from build123d import *

# Parameters (mm, degrees)
F1_DEPTH      = 1
F1_DEPTH_BACK = 1
F2_W          = 6
F2_H          = 13
F3_DEPTH      = 2
F3_DEPTH_BACK = 2
F4_R          = 5


with BuildPart() as f1:
    # F0 (on Right) → F1 (new body, two sides)
    with BuildSketch(Plane.YZ) as f1_sk:
        Polygon((-60, 5), (-60, 0), (-1, 0), (-1, 55), (1, 55), (1, 0), (60, 0), (60, 5), (7, 15), (7, 65), (4, 65), (4, 110), (-4, 110), (-4, 65), (-7, 65), (-7, 15), align=None)
    extrude(amount=F1_DEPTH)
    extrude(f1_sk.sketch, amount=-F1_DEPTH_BACK)

    # F2 (on face) → F3 (cut, two sides)
    with BuildSketch(Plane.YZ.offset(1)) as f3_sk:
        with Locations((0, 73.5)):
            Rectangle(F2_W, F2_H)
    extrude(amount=-F3_DEPTH, mode=Mode.SUBTRACT)
    extrude(f3_sk.sketch, amount=-F3_DEPTH_BACK, mode=Mode.SUBTRACT)

    # F4
    f4_edges = [f1.edges().sort_by_distance(p)[0] for p in [
        (0, -60, 5),
        (0, 60, 5),
    ]]
    fillet(f4_edges, radius=F4_R)


solid = f1.part
Could you check a few things on this model? Use its own coordinates, in mm. Give positions to 0.01 mm unless a question says otherwise; leave off trailing zeros. Order: outer loops, then holes, each group sorted by start corner. A loop starts at its lowest first (then second) coordinate and runs counter-clockwise, first axis right, second up.
Item 1: If we section it at D-D, the plane y = -41: Write out the boundary of the cut face in (x, z), plus the area to 3 significant figures.
Item 2: If we section it at A-A, the plane z = 18: Write out the boundary of the cut face in (x, y), plus the area to 3 significant figures.
Item 3: If we section it at B-B, the plane x = 0.6: Write out the boundary of the cut face in (y, z), plus the area to 3 significant figures.
Item 4: I'm going to push flat-ended pins straight in: pin 1 (1 mm diameter, centred on x = 0, z = 29.5, fed in from +Y); pin 2 (0.6 mm diameter, centred on x = 0, y = -0.5, fed in from -Z); pin 3 (1 mm diameter, centred on x = 0, z = 75, fed in from +Y). Where does each tip first touch, or does it pass through?
Item 5: I need wall thicknesses on line 1 (Y direction, x = 0.5, z = 18.5); line 2 (Y direction, x = -0.35, z = 75.5); line 3 (Y direction, x = 0.1, z = 59). Which ranges of each line are inside material? Lowest first, please.
Item 6: If we section it at C-C, the plane z = 70: Write out the boundary of the cut face in (x, y), plus the area to 3 significant figures.
Values:
1. outline: (-1, 0) - (1, 0) - (1, 8.58) - (-1, 8.58) - close
1. area: 17.2 mm2
2. outline: (-1, -7) - (1, -7) - (1, -1) - (-1, -1) - close; (-1, 1) - (1, 1) - (1, 7) - (-1, 7) - close
2. area: 24.0 mm2
3. outline: (-60, 0) - (-1, 0) - (-1, 55) - (1, 55) - (1, 0) - (60, 0) - (60, 0.86) arc R5 ccw to (55.93, 5.77) - (7, 15) - (7, 65) - (4, 65) - (4, 110) - (-4, 110) - (-4, 65) - (-7, 65) - (-7, 15) - (-55.93, 5.77) arc R5 ccw to (-60, 0.86) - close; hole (-3, 67) - (3, 67) - (3, 80) - (-3, 80) - close
3. area: 2,140 mm2
4. pin 1: stops at y = 7
4. pin 2: stops at z = 55
4. pin 3: stops at y = 4
5. line 1: y = -7 to -1, 1 to 7
5. line 2: y = -4 to -3, 3 to 4
5. line 3: y = -7 to 7
6. outline: (-1, -4) - (1, -4) - (1, -3) - (-1, -3) - close; (-1, 3) - (1, 3) - (1, 4) - (-1, 4) - close
6. area: 4.00 mm2
